from build123d import *

# Parameters (mm, degrees)
SKETCH1_W           = 17
SKETCH1_H           = 12
BOSS_EXTRUDE1_DEPTH = 1.6
SKETCH3_W           = 2.946551977
SKETCH3_H           = 5.331132701
BOSS_EXTRUDE2_DEPTH = 1.6
SKETCH10_W          = 1.272792206
SKETCH10_H          = 1.272792206
SKETCH10_H_2        = 1.272792207
BOSS_EXTRUDE3_DEPTH = 7
CHAMFER1_SIZE       = 0.25
SKETCH14_W          = 1.28426818
SKETCH14_H          = 1.28426818
SKETCH14_W_2        = 1.272792206
SKETCH14_H_2        = 1.272792206
BOSS_EXTRUDE4_DEPTH = 7
CHAMFER3_SIZE       = 0.25
FILLET1_R           = 0.1
CHAMFER4_SIZE       = 0.25
CHAMFER5_SIZE       = 1


with BuildPart() as part:
    # Sketch1 → Boss-Extrude1 (new body)
    with BuildSketch(Plane(origin=(0, 0, 0), x_dir=(1, 0, 0), z_dir=(0, 1, 0))):
        with Locations((8.5, 6)):
            Rectangle(SKETCH1_W, SKETCH1_H)
    extrude(amount=BOSS_EXTRUDE1_DEPTH)

    # Sketch3 → Boss-Extrude2 (add)
    with BuildSketch(Plane(origin=(0, 1.6, 0), x_dir=(1, 0, 0), z_dir=(0, 1, 0))):
        with Locations((9.289797438, 5.969623176)):
            Rectangle(SKETCH3_W, SKETCH3_H)
    extrude(amount=BOSS_EXTRUDE2_DEPTH)

    # Sketch5 → Revolve1 (revolve)
    with BuildSketch(Plane(origin=(15.4, 0, 0), x_dir=(0, 0, -1), z_dir=(1, 0, 0)), mode=Mode.PRIVATE) as revolve1_sk:
        with BuildLine():
            Line((2.018773021, 2.35), (2.357565231, 2.35))
            ThreePointArc((2.357565231, 2.35), (2.59682711, 1.944064718), (2.918773021, 1.6))
            Line((2.918773021, 1.6), (2.018773021, 1.6))
            Line((2.018773021, 1.6), (2.018773021, 2.35))
        make_face()
    revolve(revolve1_sk.sketch.rotate(Axis((15.4, 2.35, -2.018773021), (0, -1, 0)), 180), axis=Axis((15.4, 2.35, -2.018773021), (0, -1, 0)))

    # Sketch9 → Revolve4 (revolve)
    with BuildSketch(Plane(origin=(15.4, 0, 0), x_dir=(0, 0, -1), z_dir=(1, 0, 0)), mode=Mode.PRIVATE) as revolve4_sk:
        with BuildLine():
            Line((7.717859188, 2.35), (7.379066978, 2.35))
            Line((7.379066978, 2.35), (7.379066978, 1.6))
            Line((7.379066978, 1.6), (8.279066978, 1.6))
            ThreePointArc((8.279066978, 1.6), (7.957121066, 1.944064718), (7.717859188, 2.35))
        make_face()
    revolve(revolve4_sk.sketch.rotate(Axis((15.4, 1.6, -7.379066978), (0, -1, 0)), 180), axis=Axis((15.4, 1.6, -7.379066978), (0, -1, 0)))



with BuildPart() as body_2:
    # Sketch7 → Revolve3 (revolve)
    with BuildSketch(Plane(origin=(15.4, 0, 0), x_dir=(0, 0, -1), z_dir=(1, 0, 0)), mode=Mode.PRIVATE) as revolve3_sk:
        with BuildLine():
            Line((5.05205667, 2.35), (4.713264461, 2.35))
            Line((4.713264461, 2.35), (4.713264461, 1.6))
            Line((4.713264461, 1.6), (5.613264461, 1.6))
            ThreePointArc((5.613264461, 1.6), (5.291318549, 1.944064718), (5.05205667, 2.35))
        make_face()
    revolve(revolve3_sk.sketch.rotate(Axis((15.4, 1.6, -4.713264461), (0, -1, 0)), 180), axis=Axis((15.4, 1.6, -4.713264461), (0, -1, 0)))


with BuildPart() as part_1:
    add(part.part)

    add(body_2.part)  # Boss-Extrude3 merges body 2
    # Sketch10 → Boss-Extrude3 (add)
    with BuildSketch(Plane(origin=(0, 1.6, 0), x_dir=(1, 0, 0), z_dir=(0, 1, 0))):
        with Locations((15.4, 4.713264461)):
            Rectangle(SKETCH10_W, SKETCH10_H)
        with Locations((15.4, 2.018773021)):
            Rectangle(SKETCH10_W, SKETCH10_H_2)
        with Locations((15.4, 7.379066978)):
            Rectangle(SKETCH10_W, SKETCH10_H)
        with Locations((15.4, 10.015994476)):
            Rectangle(SKETCH10_W, SKETCH10_H)
    extrude(amount=-BOSS_EXTRUDE3_DEPTH)

    # Sketch11 → Revolve5 (revolve)
    with BuildSketch(Plane(origin=(15.4, 0, 0), x_dir=(0, 0, -1), z_dir=(1, 0, 0)), mode=Mode.PRIVATE) as revolve5_sk:
        with BuildLine():
            Line((10.283162216, 2.35), (9.944370006, 2.35))
            Line((9.944370006, 2.35), (9.944370006, 1.6))
            Line((9.944370006, 1.6), (10.844370006, 1.6))
            ThreePointArc((10.844370006, 1.6), (10.522424095, 1.944064718), (10.283162216, 2.35))
        make_face()
    revolve(revolve5_sk.sketch.rotate(Axis((15.4, 2.571627195, -9.944370006), (0, -1, 0)), 180), axis=Axis((15.4, 2.571627195, -9.944370006), (0, -1, 0)))

    # Chamfer1
    chamfer1_edges = [part_1.edges().sort_by_distance(p)[0] for p in [
        (16.036396103, -2.7, -5.349660564),
        (16.036396103, -2.7, -4.076868358),
        (14.763603897, -2.7, -4.076868358),
        (14.763603897, -2.7, -5.349660564),
        (16.036396103, -2.7, -2.655169125),
        (16.036396103, -2.7, -1.382376918),
        (14.763603897, -2.7, -1.382376918),
        (14.763603897, -2.7, -2.655169125),
        (16.036396103, -2.7, -8.015463081),
        (16.036396103, -2.7, -6.742670875),
        (14.763603897, -2.7, -6.742670875),
        (14.763603897, -2.7, -8.015463081),
        (16.036396103, -2.7, -10.652390579),
        (16.036396103, -2.7, -9.379598373),
        (14.763603897, -2.7, -9.379598373),
        (14.763603897, -2.7, -10.652390579),
    ]]
    chamfer(chamfer1_edges, length=CHAMFER1_SIZE)

    # Sketch12 → Revolve6 (revolve)
    with BuildSketch(Plane.ZY.offset(-1.5)):
        with BuildLine():
            Line((-6.967592244, 2.35), (-7.306384453, 2.35))
            Line((-7.306384453, 2.35), (-7.306384453, 1.6))
            Line((-7.306384453, 1.6), (-6.398269714, 1.6))
            ThreePointArc((-6.398269714, 1.6), (-6.7244939, 1.943449723), (-6.967592244, 2.35))
        make_face()
    revolve(axis=Axis((1.5, 2.71137522, -7.306384453), (0, -1, 0)))

    # Sketch13 → Revolve7 (revolve)
    with BuildSketch(Plane.ZY.offset(-1.5)):
        with BuildLine():
            Line((-4.274825865, 2.35), (-4.613618075, 2.35))
            Line((-4.613618075, 2.35), (-4.613618075, 1.6))
            Line((-4.613618075, 1.6), (-3.713618075, 1.6))
            ThreePointArc((-3.713618075, 1.6), (-4.035563986, 1.944064718), (-4.274825865, 2.35))
        make_face()
    revolve(axis=Axis((1.5, 2.718876296, -4.613618075), (0, -1, 0)))

    # Sketch14 → Boss-Extrude4 (add)
    with BuildSketch(Plane(origin=(0, 1.6, 0), x_dir=(1, 0, 0), z_dir=(0, 1, 0))):
        with Locations((1.5, 7.306384453)):
            Rectangle(SKETCH14_W, SKETCH14_H)
        with Locations((1.5, 4.613618075)):
            Rectangle(SKETCH14_W_2, SKETCH14_H_2)
    extrude(amount=-BOSS_EXTRUDE4_DEPTH)

    # Chamfer3
    chamfer3_edges = [part_1.edges().sort_by_distance(p)[0] for p in [
        (2.14213409, -2.7, -7.948518543),
        (2.14213409, -2.7, -6.664250363),
        (0.85786591, -2.7, -6.664250363),
        (0.85786591, -2.7, -7.948518543),
        (2.136396103, -2.7, -5.250014178),
        (2.136396103, -2.7, -3.977221972),
        (0.863603897, -2.7, -3.977221972),
        (0.863603897, -2.7, -5.250014178),
    ]]
    chamfer(chamfer3_edges, length=CHAMFER3_SIZE)

    # Fillet1
    fillet1_edges = [part_1.edges().sort_by_distance(p)[0] for p in [
        (15.4, 0, -9.379598373),
        (16.036396103, 0, -10.015994476),
        (14.763603897, 0, -10.015994476),
        (15.4, 0, -10.652390579),
        (15.4, 0, -6.742670875),
        (16.036396103, 0, -7.379066978),
        (14.763603897, 0, -7.379066978),
        (15.4, 0, -8.015463081),
        (14.763603897, 0, -4.713264461),
        (15.4, 0, -4.076868358),
        (15.4, 0, -5.349660564),
        (16.036396103, 0, -4.713264461),
        (15.4, 0, -1.382376918),
        (16.036396103, 0, -2.018773021),
        (14.763603897, 0, -2.018773021),
        (15.4, 0, -2.655169125),
        (15.911396103, 0, -9.504598373),
        (14.888603897, 0, -9.504598373),
        (14.888603897, 0, -10.527390579),
        (15.911396103, 0, -10.527390579),
        (15.911396103, 0, -6.867670875),
        (14.888603897, 0, -6.867670875),
        (14.888603897, 0, -7.890463081),
        (15.911396103, 0, -7.890463081),
        (14.888603897, 0, -4.201868358),
        (14.888603897, 0, -5.224660564),
        (15.911396103, 0, -4.201868358),
        (15.911396103, 0, -5.224660564),
        (15.911396103, 0, -1.507376918),
        (14.888603897, 0, -1.507376918),
        (14.888603897, 0, -2.530169125),
        (15.911396103, 0, -2.530169125),
        (0.85786591, 0, -7.306384453),
        (1.5, 0, -6.664250363),
        (1.5, 0, -7.948518543),
        (2.14213409, 0, -7.306384453),
        (0.863603897, 0, -4.613618075),
        (1.5, 0, -3.977221972),
        (1.5, 0, -5.250014178),
        (2.136396103, 0, -4.613618075),
        (0.98286591, 0, -6.789250363),
        (0.98286591, 0, -7.823518543),
        (2.01713409, 0, -7.823518543),
        (2.01713409, 0, -6.789250363),
        (0.988603897, 0, -4.102221972),
        (0.988603897, 0, -5.125014178),
        (2.011396103, 0, -5.125014178),
        (2.011396103, 0, -4.102221972),
    ]]
    fillet(fillet1_edges, radius=FILLET1_R)

    # Chamfer4
    chamfer4_edges = [part_1.edges().sort_by_distance(p)[0] for p in [
        (15.4, -5.4, -9.379598373),
        (16.036396103, -5.4, -10.015994476),
        (14.763603897, -5.4, -10.015994476),
        (15.4, -5.4, -10.652390579),
        (15.911396103, -5.4, -10.527390579),
        (14.888603897, -5.4, -10.527390579),
        (14.888603897, -5.4, -9.504598373),
        (15.911396103, -5.4, -9.504598373),
        (15.4, -5.4, -6.742670875),
        (16.036396103, -5.4, -7.379066978),
        (14.763603897, -5.4, -7.379066978),
        (15.4, -5.4, -8.015463081),
        (15.911396103, -5.4, -7.890463081),
        (14.888603897, -5.4, -7.890463081),
        (14.888603897, -5.4, -6.867670875),
        (15.911396103, -5.4, -6.867670875),
        (14.763603897, -5.4, -4.713264461),
        (15.4, -5.4, -4.076868358),
        (16.036396103, -5.4, -4.713264461),
        (15.4, -5.4, -5.349660564),
        (15.911396103, -5.4, -5.224660564),
        (15.911396103, -5.4, -4.201868358),
        (14.888603897, -5.4, -5.224660564),
        (14.888603897, -5.4, -4.201868358),
        (15.4, -5.4, -1.382376918),
        (16.036396103, -5.4, -2.018773021),
        (14.763603897, -5.4, -2.018773021),
        (15.4, -5.4, -2.655169125),
        (15.911396103, -5.4, -2.530169125),
        (14.888603897, -5.4, -2.530169125),
        (14.888603897, -5.4, -1.507376918),
        (15.911396103, -5.4, -1.507376918),
        (0.85786591, -5.4, -7.306384453),
        (1.5, -5.4, -6.664250363),
        (2.14213409, -5.4, -7.306384453),
        (1.5, -5.4, -7.948518543),
        (2.01713409, -5.4, -6.789250363),
        (2.01713409, -5.4, -7.823518543),
        (0.98286591, -5.4, -7.823518543),
        (0.98286591, -5.4, -6.789250363),
        (0.863603897, -5.4, -4.613618075),
        (1.5, -5.4, -3.977221972),
        (2.136396103, -5.4, -4.613618075),
        (1.5, -5.4, -5.250014178),
        (2.011396103, -5.4, -4.102221972),
        (2.011396103, -5.4, -5.125014178),
        (0.988603897, -5.4, -5.125014178),
        (0.988603897, -5.4, -4.102221972),
    ]]
    chamfer(chamfer4_edges, length=CHAMFER4_SIZE)

    # Chamfer5
    chamfer5_edges = [part_1.edges().sort_by_distance(p)[0] for p in [
        (0, 0.8, -12),
        (0, 0.8, 0),
        (17, 0.8, 0),
        (17, 0.8, -12),
    ]]
    chamfer(chamfer5_edges, length=CHAMFER5_SIZE)


solid = part_1.part
Here's how the part is built. I have some questions about the finished solid (model axes, mm). A direction names the side the tool comes from. Give positions to 0.01 mm unless a question says otherwise; leave off trailing zeros. Order: outer loops, then holes, each group sorted by start corner. A loop starts at its lowest first (then second) coordinate and runs counter-clockwise, first axis right, second up. Notation, with made-up numbers: (-1.5, 30.5) -> (6.5, 30.5) arc R21 cw to (6.5, 54.5) -> close; hole circle Ø6 at (27.5, -15). An arc over 180 degrees is marked (long way). One line per item, written item: value. Start each with the question number.
1. For faces 1 (the face through (9, 2, -3.304)), 2 (the face through (7.817, 2, -6)), 3 (the face through (6, 1.6, -6)), 4 (the face through (9, 2, -8.635)), which set-ups out of +Z, -Z, +X, -X, +Y, -Y let a thin tool reach every point of the face, with its end or its side?
2. Imagine slicing it at B-B, the plane x = 10. List the corners of the cut face in (y, z) for me.
3. Will these pins go through, and if not, where does the flat tip stop? pin 1 Ø1.5 at (x, z) = (7.5, -2.5) entering from -Y; pin 2 Ø0.9 at (x, y) = (1.5, -3) entering from +Z; pin 3 Ø0.6 at (y, z) = (-3, -10) entering from -X; pin 4 Ø5 at (y, z) = (2, -6.5) entering from +X.
4. We'd pull the mould along X, two halves only. Please class faces 5 (the face through (9, 3.2, -6)), 6 (the face through (16.5, 0.8, -0.5)), 7 (the face through (10.763, 2, -6)): released by +X, released by -X, zero draft, split by the parting line, or undercut.
5. Imagine slicing it at A-A, the plane y = -3.5. Count the separate pieces of the cut face and the enclosed holes in it, plus the area to 3 significant figures.
6. I need wall thicknesses on probe 1 along Z at (x, y) = (15.5, -0.25); probe 2 along Z at (x, y) = (1.5, -0.5); probe 3 along Y at (x, z) = (10.5, -9). Which ranges of each line are inside material? Lowest first, please. Write a range as from..to.
7. Imagine slicing it at C-C, the plane x = 7.25. List the corners of the cut face in (y, z) for me.
Values follow:
1. face 1: +Z, +X, -X, +Y
1. face 2: +Z, -Z, +Y
1. face 3: +Y
1. face 4: -Z, +X, -X, +Y
2. outline: (0, -12) -> (1.6, -12) -> (1.6, -8.64) -> (3.2, -8.64) -> (3.2, -3.3) -> (1.6, -3.3) -> (1.6, 0) -> (0, 0) -> close
3. pin 1: stops at y = 0
3. pin 2: stops at z = -3.98
3. pin 3: stops at x = 14.76
3. pin 4: stops at x = 17
4. face 5: zero draft
4. face 6: released by +X
4. face 7: undercut
5. separate pieces: 6
5. enclosed holes: 0
5. area: 9.00 mm2
6. probe 1: z = -10.65..-9.38, -8.02..-6.74, -5.35..-4.08, -2.66..-1.38
6. probe 2: z = -7.95..-6.66, -5.25..-3.98
6. probe 3: y = 0..1.6
7. outline: (0, -12) -> (1.6, -12) -> (1.6, 0) -> (0, 0) -> close
